```python
from build123d import *

# Parameters (mm, degrees)
BOSS_EXTRUDE1_DEPTH                             = 100
CSK_FOR_M4_FLAT_HEAD_MACHINE_SCREW1_D           = 4.5
CSK_FOR_M4_FLAT_HEAD_MACHINE_SCREW1_CSINK_D     = 9.4
CSK_FOR_M4_FLAT_HEAD_MACHINE_SCREW1_CSINK_ANGLE = 90
CSK_FOR_M4_FLAT_HEAD_MACHINE_SCREW4_D           = 4.5
CSK_FOR_M4_FLAT_HEAD_MACHINE_SCREW4_CSINK_D     = 9.4
CSK_FOR_M4_FLAT_HEAD_MACHINE_SCREW4_CSINK_ANGLE = 90


with BuildPart() as part:
    # Sketch1 → Boss-Extrude1 (new body)
    with BuildSketch(Plane.XY):
        with BuildLine():
            Line((0, 40), (0, 16.35))
            ThreePointArc((0, 16.35), (4.788804128, 4.788804128), (16.35, 0))
            Line((16.35, 0), (40, 0))
            Line((40, 0), (40, 6.35))
            Line((40, 6.35), (16.35, 6.35))
            ThreePointArc((16.35, 6.35), (9.278932188, 9.278932188), (6.35, 16.35))
            Line((6.35, 16.35), (6.35, 40))
            Line((6.35, 40), (0, 40))
        make_face()
    extrude(amount=BOSS_EXTRUDE1_DEPTH)

    # CSK for M4 Flat Head Machine Screw1 (through all)
    with Locations(Plane(origin=(0, 6.35, 0), x_dir=(1, 0, 0), z_dir=(0, 1, 0))):
        with Locations((30, -90), (30, -50), (30, -10)):
            CounterSinkHole(CSK_FOR_M4_FLAT_HEAD_MACHINE_SCREW1_D / 2, CSK_FOR_M4_FLAT_HEAD_MACHINE_SCREW1_CSINK_D / 2, counter_sink_angle=CSK_FOR_M4_FLAT_HEAD_MACHINE_SCREW1_CSINK_ANGLE)

    # CSK for M4 Flat Head Machine Screw4 (through all)
    with Locations(Plane(origin=(6.35, 0, 0), x_dir=(0, -1, 0), z_dir=(1, 0, 0))):
        with Locations((-30, -90), (-30, -50), (-30, -10)):
            CounterSinkHole(CSK_FOR_M4_FLAT_HEAD_MACHINE_SCREW4_D / 2, CSK_FOR_M4_FLAT_HEAD_MACHINE_SCREW4_CSINK_D / 2, counter_sink_angle=CSK_FOR_M4_FLAT_HEAD_MACHINE_SCREW4_CSINK_ANGLE)


solid = part.part
```
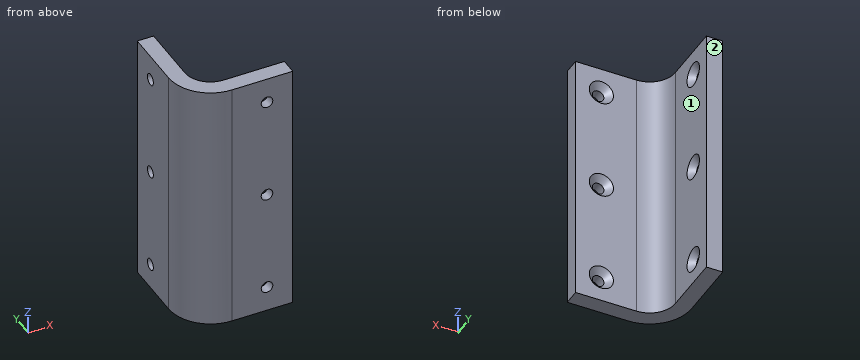
Model file for the job. Use its own axes, mm. Face numbers are marked on the shaded views. A direction names the side the tool comes from. Round coordinates to 2 decimals unless told otherwise and drop trailing zeros. Write each loop counter-clockwise with the first axis right and the second up, starting at its lowest first coordinate (ties: lowest second). Pieces come first, ordered by that corner, then holes. Notation, with made-up numbers: (33, 72) - (72, 72) arc R14 ccw to (72, 95) - close; hole circle Ø4 at (22, 12.25). An arc over 180 degrees is marked (long way). Use CSV: the item, a comma, the result in double quotes. Start each with the question number.
Item 1: Tool access for the marked faces 1 and 2: list every direction of +Z, -Z, +X, -X, +Y, -Y with a clear straight run to the whole face (end or side of a thin tool).
Item 2: Band-saw the part on B-B (y = 30). Write the cut outline in (x, z), and give its area (3 significant figures).
Item 3: Band-saw the part on D-D (z = 78). Write the cut outline in (x, y), and give its area (3 significant figures).
Item 4: Pin check, flat tips, straight feed: P1, Ø6, axis at x = 30, z = 90, coming from the -Y side; P2, Ø19, axis at y = 33, z = 73.5, coming from the +X side; P3, Ø7, axis at x = 30, z = 50, coming from the +Y side; P4, Ø3.5, axis at x = 30, z = 10, coming from the -Y side. Stop position of each tip, or through.
Item 5: Band-saw the part on A-A (z = 50). Write the cut outline in (x, y).
Item 6: Drill centre lines: L1, parallel to Z at x = 2, y = 30; L2, parallel to Y at x = 25, z = 68.5. Where is each one in solid material? Low to high. Write a range as [from, to].
Checked values:
1,face 1,"+Z, -Z, +X, +Y"
1,face 2,"+Z, -Z, +X, -X, +Y"
2,outline,"(0, 0) - (6.35, 0) - (6.35, 5.3) - (3.9, 7.75) - (0, 7.75) - close; (0, 12.25) - (3.9, 12.25) - (6.35, 14.7) - (6.35, 45.3) - (3.9, 47.75) - (0, 47.75) - close; (0, 52.25) - (3.9, 52.25) - (6.35, 54.7) - (6.35, 85.3) - (3.9, 87.75) - (0, 87.75) - close; (0, 92.25) - (3.9, 92.25) - (6.35, 94.7) - (6.35, 100) - (0, 100) - close"
2,area,"531 mm²"
3,outline,"(0, 16.35) arc R16.35 ccw to (16.35, 0) - (40, 0) - (40, 6.35) - (16.35, 6.35) arc R10 cw to (6.35, 16.35) - (6.35, 40) - (0, 40) - close"
3,area,"432 mm²"
4,P1,"stops at y = 0"
4,P2,"stops at x = 6.35"
4,P3,"stops at y = 5.15"
4,P4,"passes through"
5,outline,"(0, 16.35) arc R16.35 ccw to (16.35, 0) - (27.75, 0) - (27.75, 3.9) - (25.3, 6.35) - (16.35, 6.35) arc R10 cw to (6.35, 16.35) - (6.35, 25.3) - (3.9, 27.75) - (0, 27.75) - close; (0, 32.25) - (3.9, 32.25) - (6.35, 34.7) - (6.35, 40) - (0, 40) - close; (32.25, 0) - (40, 0) - (40, 6.35) - (34.7, 6.35) - (32.25, 3.9) - close"
6,L1,"z = [0, 7.75], [12.25, 47.75], [52.25, 87.75], [92.25, 100]"
6,L2,"y = [0, 6.35]"
